Model file for the job. Use its own axes, mm. Face numbers are marked on the shaded views. Give positions to 0.01 mm unless a question says otherwise; leave off trailing zeros. Use CSV: the item, a comma, the result in double quotes.
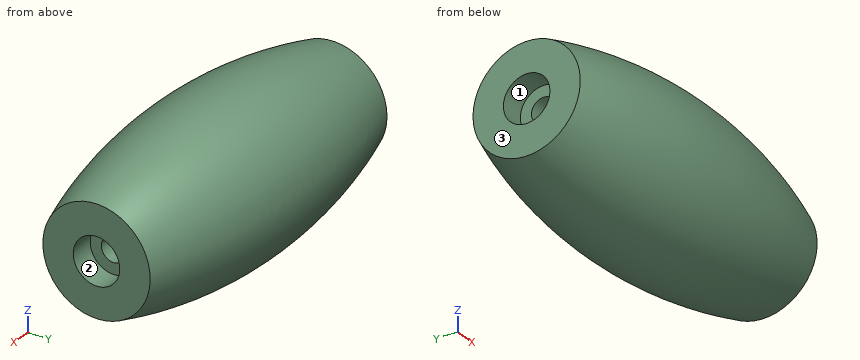
from build123d import *

# Parameters (mm, degrees)
CBORE_FOR_M3_HEX_SOCKET_HEAD_CAP_SCREW1_D           = 3.4
CBORE_FOR_M3_HEX_SOCKET_HEAD_CAP_SCREW1_DEPTH       = 11.57
CBORE_FOR_M3_HEX_SOCKET_HEAD_CAP_SCREW1_CBORE_D     = 6.5
CBORE_FOR_M3_HEX_SOCKET_HEAD_CAP_SCREW1_CBORE_DEPTH = 3.4
CBORE_FOR_M3_HEX_SOCKET_HEAD_CAP_SCREW1_TIP         = 1.021463052
CBORE_FOR_M3_HEX_SOCKET_HEAD_CAP_SCREW2_D           = 3.4
CBORE_FOR_M3_HEX_SOCKET_HEAD_CAP_SCREW2_DEPTH       = 11.57
CBORE_FOR_M3_HEX_SOCKET_HEAD_CAP_SCREW2_CBORE_D     = 6.5
CBORE_FOR_M3_HEX_SOCKET_HEAD_CAP_SCREW2_CBORE_DEPTH = 3.4
CBORE_FOR_M3_HEX_SOCKET_HEAD_CAP_SCREW2_TIP         = 1.021463052


with BuildPart() as part:
    # Sketch1 → Revolve1 (revolve)
    with BuildSketch(Plane.XY):
        with BuildLine():
            Line((0, 0), (0, 7.5))
            ThreePointArc((0, 7.5), (23.75, 11.106692047), (47.5, 7.5))
            Line((47.5, 7.5), (47.5, 0))
            Line((47.5, 0), (0, 0))
        make_face()
    revolve(axis=Axis((47.5, 0, 0), (-1, 0, 0)))

    # CBORE for M3 Hex Socket Head Cap Screw1
    with Locations(Plane(origin=(47.5, 0, 0), x_dir=(0, 0, -1), z_dir=(1, 0, 0))):
        with Locations((0, 0)):
            CounterBoreHole(CBORE_FOR_M3_HEX_SOCKET_HEAD_CAP_SCREW1_D / 2, CBORE_FOR_M3_HEX_SOCKET_HEAD_CAP_SCREW1_CBORE_D / 2, CBORE_FOR_M3_HEX_SOCKET_HEAD_CAP_SCREW1_CBORE_DEPTH, depth=CBORE_FOR_M3_HEX_SOCKET_HEAD_CAP_SCREW1_DEPTH)
            with Locations((0, 0, -(CBORE_FOR_M3_HEX_SOCKET_HEAD_CAP_SCREW1_DEPTH + CBORE_FOR_M3_HEX_SOCKET_HEAD_CAP_SCREW1_TIP / 2))):  # 118° drill point
                Cone(0, CBORE_FOR_M3_HEX_SOCKET_HEAD_CAP_SCREW1_D / 2, CBORE_FOR_M3_HEX_SOCKET_HEAD_CAP_SCREW1_TIP, mode=Mode.SUBTRACT)

    # CBORE for M3 Hex Socket Head Cap Screw2
    with Locations(Plane.ZY):
        with Locations((0, 0)):
            CounterBoreHole(CBORE_FOR_M3_HEX_SOCKET_HEAD_CAP_SCREW2_D / 2, CBORE_FOR_M3_HEX_SOCKET_HEAD_CAP_SCREW2_CBORE_D / 2, CBORE_FOR_M3_HEX_SOCKET_HEAD_CAP_SCREW2_CBORE_DEPTH, depth=CBORE_FOR_M3_HEX_SOCKET_HEAD_CAP_SCREW2_DEPTH)
            with Locations((0, 0, -(CBORE_FOR_M3_HEX_SOCKET_HEAD_CAP_SCREW2_DEPTH + CBORE_FOR_M3_HEX_SOCKET_HEAD_CAP_SCREW2_TIP / 2))):  # 118° drill point
                Cone(0, CBORE_FOR_M3_HEX_SOCKET_HEAD_CAP_SCREW2_D / 2, CBORE_FOR_M3_HEX_SOCKET_HEAD_CAP_SCREW2_TIP, mode=Mode.SUBTRACT)


solid = part.part
(1) Pull direction Y, two halves, no side cores. Call the marked faces 1, 2 and 3: released by +Y, released by -Y, zero draft, split by the parting line, or undercut.
Checked values:
face 1,"undercut"
face 2,"undercut"
face 3,"zero draft"
(2) Flat gauge pins, fed straight in: P1, Ø4.5, axis at y = 0, z = 0, coming from the +X side; P2, Ø8, axis at x = 41.5, z = -1.5, coming from the -Y side; P3, Ø6, axis at y = 0, z = 0, coming from the -X side. Where does each tip first touch, or does it go through?
Checked values:
P1,"stops at x = 44.1"
P2,"stops at y = -9.88"
P3,"stops at x = 3.4"
(3) Wall check: probe 1 along Z at (x, y) = (7, 0.5); probe 2 along Y at (x, z) = (7.5, 0); probe 3 along Y at (x, z) = (5.25, 0). Give the ranges that are in metal, low to high. Write a range as [from, to].
Checked values:
probe 1,"z = [-9.32, -1.62], [1.62, 9.32]"
probe 2,"y = [-9.44, -1.7], [1.7, 9.44]"
probe 3,"y = [-8.94, -1.7], [1.7, 8.94]"
